Design review of the part built by this model. Coordinates are the model's own, in mm. A direction names the side the tool comes from. Give positions to 0.01 mm unless a question says otherwise; leave off trailing zeros. Write each question's results on one line, items separated by ' | '. Start each with the question number.
(1) Clearance check with flat-ended pins moving along their axes: pin 1 (3 mm diameter, centred on x = -17.5, y = 16.5, fed in from +Z); pin 2 (5 mm diameter, centred on x = -5.5, y = 5.5, fed in from +Z); pin 3 (6 mm diameter, centred on y = 6.5, z = -12, fed in from +X); pin 4 (5.5 mm diameter, centred on x = 21.65, z = 12.5, fed in from +Y). State where each tip first meets the part, or that it passes through.
(2) For faces 1 (the face through (0.08, 1.48, -8.2)), 2 (the face through (-17.31, 11.51, 15.27)), 3 (the face through (-24.58, 2.38, 11.85)), list the 3-axis set-ups (+Z, -Z, +X, -X, +Y, -Y) from which the entire face can be reached by the end or side of a thin tool; tool diameter is ignored.
(3) Take a section at A-A (y = 11.25). Count the separate pieces of the cut face and the enclosed holes in it, plus the area to 3 significant figures.
(4) To check wall thickness, follow probe 1 along X at (y, z) = (10.5, 0); probe 2 along X at (y, z) = (10.5, 6); probe 3 along X at (y, z) = (4.25, 0). State the ranges of each line that lie inside material, in increasing order.
(5) Mouldability with a two-part tool opening along Z and no side actions: class faces 4 (the face through (-3, 9, 3)), 5 (the face through (-31.24, 10.38, -6.94)) as released by +Z, released by -Z, zero draft, split by the parting line, or undercut.
from build123d import *

# Parameters (mm, degrees)
SKETCH_1_R          = 32
SKETCH_1_R_2        = 4
SKETCH_1_R_3        = 3
EXTRUDE_1_DEPTH     = 19
FILLET_1_R          = 2
SKETCH_2_R          = 5.15
CUT_EXTRUDE_1_DEPTH = 15.2
SKETCH_3_R          = 2.55
CUT_EXTRUDE_2_DEPTH = 15
SKETCH_4_R          = 1.1
CUT_EXTRUDE_3_DEPTH = 50.081564832
SKETCH_7_R          = 1.8
CUT_EXTRUDE_5_DEPTH = 3
CHAMFER_1_SIZE      = 1
SKETCH_8_R          = 7.1
CUT_EXTRUDE_6_DEPTH = 10
SKETCH_9_R          = 0.9
CUT_EXTRUDE_7_DEPTH = 50.081564832


with BuildPart() as part:
    # Эскиз1 → Бобышка-Вытянуть1 (new body)
    with BuildSketch(Plane(origin=(0, 0, 0), x_dir=(1, 0, 0), z_dir=(0, 1, 0))):
        with Locations(Location((0, 0, 0), (0, 0, 270))):
            Circle(SKETCH_1_R)
        with Locations(Location((0, 0, 0), (0, 0, 270))):
            Circle(SKETCH_1_R_2, mode=Mode.SUBTRACT)
        with Locations(Location((0, 25, 0), (0, 0, 270))):
            Circle(SKETCH_1_R_3, mode=Mode.SUBTRACT)
        with Locations(Location((21.650635095, -12.5, 0), (0, 0, 270))):
            Circle(SKETCH_1_R_3, mode=Mode.SUBTRACT)
        with Locations(Location((-21.650635095, -12.5, 0), (0, 0, 270))):
            Circle(SKETCH_1_R_3, mode=Mode.SUBTRACT)
    extrude(amount=EXTRUDE_1_DEPTH)

    # Скругление1
    fillet_1_edges = [part.edges().sort_by_distance(p)[0] for p in [
        (0, 0, -32),
    ]]
    fillet(fillet_1_edges, radius=FILLET_1_R)

    # Эскиз2 → Вырез-Вытянуть1 (cut)
    with BuildSketch(Plane(origin=(0, 19, 0), x_dir=(1, 0, 0), z_dir=(0, 1, 0))):
        with Locations(Location((0, 25, 0), (0, 0, 270))):
            Circle(SKETCH_2_R)
        with Locations(Location((21.650635095, -12.5, 0), (0, 0, 270))):
            Circle(SKETCH_2_R)
        with Locations(Location((-21.650635095, -12.5, 0), (0, 0, 270))):
            Circle(SKETCH_2_R)
    extrude(amount=-CUT_EXTRUDE_1_DEPTH, mode=Mode.SUBTRACT)

    # Эскиз3 → Вырез-Вытянуть2 (cut)
    with BuildSketch(Plane.XZ):
        with Locations(Location((0, 25, 0), (0, 0, 270))):
            Circle(SKETCH_3_R)
        with Locations(Location((21.650635095, -12.5, 0), (0, 0, 270))):
            Circle(SKETCH_3_R)
        with Locations(Location((-21.650635095, -12.5, 0), (0, 0, 270))):
            Circle(SKETCH_3_R)
    extrude(amount=-CUT_EXTRUDE_2_DEPTH, mode=Mode.SUBTRACT)

    # Эскиз4 → Вырез-Вытянуть3 (cut, through all)
    with BuildSketch(Plane(origin=(0, 19, 0), x_dir=(1, 0, 0), z_dir=(0, 1, 0))):
        with Locations(Location((0, 10, 0), (0, 0, 270))):
            Circle(SKETCH_4_R)
        with Locations(Location((8.660254038, 5, 0), (0, 0, 270))):
            Circle(SKETCH_4_R)
        with Locations(Location((8.660254038, -5, 0), (0, 0, 270))):
            Circle(SKETCH_4_R)
        with Locations(Location((0, -10, 0), (0, 0, 270))):
            Circle(SKETCH_4_R)
        with Locations(Location((-8.660254038, -5, 0), (0, 0, 270))):
            Circle(SKETCH_4_R)
        with Locations(Location((-8.660254038, 5, 0), (0, 0, 270))):
            Circle(SKETCH_4_R)
    extrude(amount=-CUT_EXTRUDE_3_DEPTH, mode=Mode.SUBTRACT)

    # Эскиз7 → Вырез-Вытянуть5 (cut)
    with BuildSketch(Plane.XZ):
        with Locations(Location((8.660254038, 5, 0), (0, 0, 270))):
            Circle(SKETCH_7_R)
        with Locations(Location((0, -10, 0), (0, 0, 270))):
            Circle(SKETCH_7_R)
        with Locations(Location((-8.660254038, 5, 0), (0, 0, 270))):
            Circle(SKETCH_7_R)
    extrude(amount=-CUT_EXTRUDE_5_DEPTH, mode=Mode.SUBTRACT)

    # Фаска1
    chamfer_1_edges = [part.edges().sort_by_distance(p)[0] for p in [
        (21.650635095, 0, 9.5),
        (-21.650635095, 0, 9.5),
        (0, 0, 27.55),
        (21.650635095, 0, -9.95),
        (-21.650635095, 0, -9.95),
        (0, 0, -4),
        (0, 0, -28),
    ]]
    chamfer(chamfer_1_edges, length=CHAMFER_1_SIZE)

    # Эскиз8 → Вырез-Вытянуть6 (cut)
    with BuildSketch(Plane(origin=(0, 19, 0), x_dir=(1, 0, 0), z_dir=(0, 1, 0))):
        with Locations(Location((0, 0, 0), (0, 0, 270))):
            Circle(SKETCH_8_R)
    extrude(amount=-CUT_EXTRUDE_6_DEPTH, mode=Mode.SUBTRACT)

    # Эскиз9 → Вырез-Вытянуть7 (cut, through all)
    with BuildSketch(Plane(origin=(0, 19, 0), x_dir=(1, 0, 0), z_dir=(0, 1, 0))):
        with Locations(Location((-8, 23.685438565, 0), (0, 0, 270))):
            Circle(SKETCH_9_R)
        with Locations(Location((8, 23.685438565, 0), (0, 0, 270))):
            Circle(SKETCH_9_R)
        with Locations(Location((16.512191497, -18.770922513, 0), (0, 0, 270))):
            Circle(SKETCH_9_R)
        with Locations(Location((24.512191497, -4.914516052, 0), (0, 0, 270))):
            Circle(SKETCH_9_R)
        with Locations(Location((-24.512191497, -4.914516052, 0), (0, 0, 270))):
            Circle(SKETCH_9_R)
        with Locations(Location((-16.512191497, -18.770922513, 0), (0, 0, 270))):
            Circle(SKETCH_9_R)
    extrude(amount=-CUT_EXTRUDE_7_DEPTH, mode=Mode.SUBTRACT)


solid = part.part
Report:
1) pin 1: z = 27.71 | pin 2: z = 31.86 | pin 3: x = 30.71 | pin 4: through
2) face 1: -Y | face 2: +Y | face 3: +Y, -Y
3) separate pieces: 1 | enclosed holes: 19 | area: 2,710 mm2
4) probe 1: -32 to -7.1, 7.1 to 32 | probe 2: -31.43 to -9.12, -8.2 to -3.8, 3.8 to 8.2, 9.12 to 31.43 | probe 3: -32 to -4, 4 to 32
5) face 4: undercut | face 5: split by the parting line
